```python
from build123d import *

# Parameters (mm, degrees)
F1_DEPTH = 12.7
F2_W     = 31.30851
F2_H     = 20.404518
F3_DEPTH = 50.8
F5_DEPTH = 25.4
F7_DEPTH = 12.7


with BuildPart() as f1:
    # F0 (on Top) → F1 (new body)
    with BuildSketch(Plane.XY):
        with BuildLine():
            Line((-15.654255, -20.404518), (15.654255, -20.404518))
            Line((15.654255, -20.404518), (15.654255, 20.404518))
            ThreePointArc((15.654255, 20.404518), (0, 36.058772), (-15.654255, 20.404518))
            Line((-15.654255, 20.404518), (-15.654255, -20.404518))
        make_face()
    extrude(amount=F1_DEPTH)

    # F2 (on face) → F3 (join)
    with BuildSketch(Plane.XY.offset(12.7)):
        with Locations((0, -10.202259)):
            Rectangle(F2_W, F2_H)
    extrude(amount=F3_DEPTH)

    # F4 (on face) → F5 (cut)
    with BuildSketch(Plane(origin=(0, 0, 0), x_dir=(-1, 0, 0), z_dir=(0, 1, 0))):
        with BuildLine():
            Line((6.924376, 63.5), (-6.511585, 63.5))
            Line((-6.511585, 63.5), (-6.511585, 32.147441))
            ThreePointArc((-6.511585, 32.147441), (0.206395, 25.42946), (6.924376, 32.147441))
            Line((6.924376, 32.147441), (6.924376, 63.5))
        make_face()
    extrude(amount=-F5_DEPTH, mode=Mode.SUBTRACT)

    # F6 (on face) → F7 (cut)
    with BuildSketch(Plane(origin=(-15.654255, 0, 0), x_dir=(0, -1, 0), z_dir=(-1, 0, 0))):
        Polygon((0, 12.7), (-10.202259, 12.7), (-10.202259, 0), (20.404518, 0), (20.404518, 12.7), (20.404518, 21.397056), (0, 21.397056), align=None)
    extrude(amount=-F7_DEPTH, mode=Mode.SUBTRACT)


solid = f1.part
```
Could you check a few things on this model? Use its own coordinates, in mm. A direction names the side the tool comes from. Round coordinates to 2 decimals unless told otherwise and drop trailing zeros. Write each loop counter-clockwise with the first axis right and the second up, starting at its lowest first coordinate (ties: lowest second). Pieces come first, ordered by that corner, then holes. Notation, with made-up numbers: M 43.5,85 L 79.5,85 A19 ccw 79.5,89 Z; hole C 21,8 d5. An arc over 180 degrees is marked long. Answer in a Markdown table with one row per item. Add a question column.
Q1. Imagine slicing it at C-C (y = -13.5). Please give me the cut outline in (x, z).
Q2. Imagine slicing it at B-B (x = -11.5). Please give me the cut outline in (y, z).
Q3. If I drill on line 1 (X direction, y = -12.5, z = 45); line 2 (Y direction, x = -2.5, z = 23); line 3 (Z direction, x = 10, y = 24.5), over which ranges is the centre line in solid material (lowest first)? Write a range as from..to.
Q4. Imagine slicing it at A-A (z = 60). Please give me the cut outline in (x, y).
Q5. Imagine slicing it at D-D (z = 8). Please give me the cut outline in (x, y).
Q6. If we mould it in two halves opening along X, with no side actions, what happens to faces 1 (the flat face through (6.512, -10, 48)), 2 (the flat face through (15.654, -5, 24)), 3 (the cylindrical face through (-0.06, -10.06, 25.43)), 4 (the flat face through (-9, 10.202, 6))? For each: +X half, -X half, draft (parallel to the pull), parting line (faces both ways), or undercut.
Q7. Will these pins go through, and if not, where does the flat tip stop? pin 1 Ø2 at (x, z) = (7, 54) entering from +Y; pin 2 Ø10.5 at (y, z) = (-9.5, 14.5) entering from -X; pin 3 Ø9.5 at (x, y) = (-3.5, 25.5) entering from +Z.
Q8. On a 3-axis mill with a long thin cutter (end or side, diameter ignored), from which of +Z, -Z, +X, -X, +Y, -Y can I reach the whole of each face in a straight line? I mean faces 5 (the flat face through (-2.954, -8, 11)), 6 (the flat face through (0, 18, 12.7)), 7 (the flat face through (-6.924, -10, 48)), 8 (the flat face through (-9, -10, 21.397)). Say none if no direction works.
Values:
| question | item | result |
|---|---|---|
| 1 | outline | M -15.65,21.4 L -2.95,21.4 L -2.95,0 L 15.65,0 L 15.65,63.5 L 6.51,63.5 L 6.51,32.15 A6.72 cw -6.92,32.15 L -6.92,63.5 L -15.65,63.5 Z |
| 2 | outline | M -20.4,21.4 L 0,21.4 L 0,63.5 L -20.4,63.5 Z; M 10.2,0 L 31.03,0 L 31.03,12.7 L 10.2,12.7 Z |
| 3 | line 1 | -15.65..-6.92, 6.51..15.65 |
| 3 | line 2 | -20.4..0 |
| 3 | line 3 | 0..12.7 |
| 4 | outline | M -15.65,-20.4 L -6.92,-20.4 L -6.92,0 L -15.65,0 Z; M 6.51,-20.4 L 15.65,-20.4 L 15.65,0 L 6.51,0 Z |
| 5 | outline | M -15.65,10.2 L -2.95,10.2 L -2.95,-20.4 L 15.65,-20.4 L 15.65,20.4 A15.65 ccw -15.65,20.4 Z |
| 6 | face 1 | undercut |
| 6 | face 2 | +X half |
| 6 | face 3 | undercut |
| 6 | face 4 | draft |
| 7 | pin 1 | y = 0 |
| 7 | pin 2 | x = -2.95 |
| 7 | pin 3 | z = 12.7 |
| 8 | face 5 | -Z, -X, -Y |
| 8 | face 6 | +Z, +X, -X, +Y |
| 8 | face 7 | +Z, +Y, -Y |
| 8 | face 8 | -Z, -X, +Y, -Y |
